from build123d import *

# Parameters (mm, degrees)
BOSS_EXTRUDE1_DEPTH = 5.08
SKETCH3_W           = 12.7
SKETCH3_H           = 12.7
SKETCH3_H_2         = 12.575411903
SKETCH3_W_2         = 12.822150439
CUT_EXTRUDE1_DEPTH  = 114.705788771


with BuildPart() as part:
    # Sketch2 → Boss-Extrude1 (new body)
    with BuildSketch(Plane(origin=(0, 0, 0), x_dir=(1, 0, 0), z_dir=(0, 1, 0))):
        with BuildLine():
            Line((-88.9, -50.8), (88.9, -50.8))
            ThreePointArc((88.9, -50.8), (97.880256121, -47.080256121), (101.6, -38.1))
            Line((101.6, -38.1), (101.6, 38.1))
            ThreePointArc((101.6, 38.1), (97.880256121, 47.080256121), (88.9, 50.8))
            Line((88.9, 50.8), (-88.9, 50.8))
            ThreePointArc((-88.9, 50.8), (-97.880256121, 47.080256121), (-101.6, 38.1))
            Line((-101.6, 38.1), (-101.6, -38.1))
            ThreePointArc((-101.6, -38.1), (-97.880256121, -47.080256121), (-88.9, -50.8))
        make_face()
    extrude(amount=BOSS_EXTRUDE1_DEPTH)

    # Sketch3 → Cut-Extrude1 (cut, through all)
    with BuildSketch(Plane(origin=(0, 5.08, 0), x_dir=(1, 0, 0), z_dir=(0, 1, 0))):
        with Locations((-69.838651623, -44.45)):
            Rectangle(SKETCH3_W, SKETCH3_H)
        with Locations((-69.838651623, 44.512294049)):
            Rectangle(SKETCH3_W, SKETCH3_H_2)
        with Locations((69.673417763, -44.45)):
            Rectangle(SKETCH3_W_2, SKETCH3_H)
        with Locations((69.673417763, 44.512294049)):
            Rectangle(SKETCH3_W_2, SKETCH3_H_2)
    extrude(amount=-CUT_EXTRUDE1_DEPTH, mode=Mode.SUBTRACT)


solid = part.part
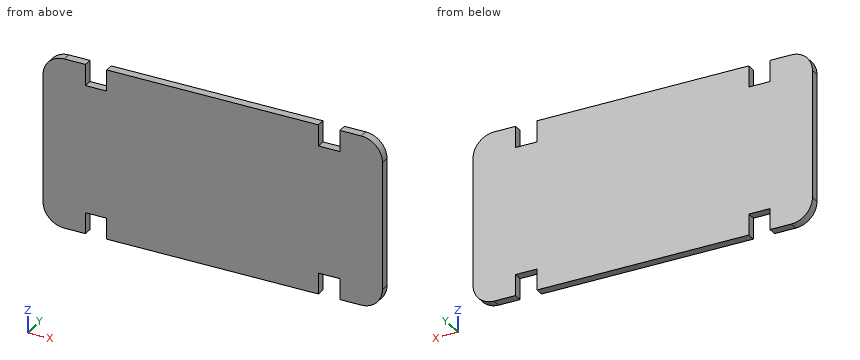
Could you check a few things on this model? Use its own coordinates, in mm. Round coordinates to 2 decimals unless told otherwise and drop trailing zeros. Order: outer loops, then holes, each group sorted by start corner. A loop starts at its lowest first (then second) coordinate and runs counter-clockwise, first axis right, second up.
Q1. Imagine slicing it at B-B, the plane x = 68. List the corners of the cut face in (y, z) for me.
Geometry says:
outline: (0, -38.22) - (5.08, -38.22) - (5.08, 38.1) - (0, 38.1) - close
Q2. Please list where these lines run through material, in increasing order: probe 1 along X at (y, z) = (4.3, -39.5); probe 2 along X at (y, z) = (0.4, 43); probe 3 along Z at (x, y) = (-89.5, 0.6).
Geometry says:
probe 1: x = -101.52 to -76.19, -63.49 to 63.26, 76.08 to 101.52
probe 2: x = -100.62 to -76.19, -63.49 to 63.26, 76.08 to 100.62
probe 3: z = -50.79 to 50.79
Q3. Imagine slicing it at A-A, the plane y = 3.5. List the corners of the cut face in (x, z) for me.
Geometry says:
outline: (-101.6, -38.1) arc R12.7 ccw to (-88.9, -50.8) - (-76.19, -50.8) - (-76.19, -38.22) - (-63.49, -38.22) - (-63.49, -50.8) - (63.26, -50.8) - (63.26, -38.22) - (76.08, -38.22) - (76.08, -50.8) - (88.9, -50.8) arc R12.7 ccw to (101.6, -38.1) - (101.6, 38.1) arc R12.7 ccw to (88.9, 50.8) - (76.08, 50.8) - (76.08, 38.1) - (63.26, 38.1) - (63.26, 50.8) - (-63.49, 50.8) - (-63.49, 38.1) - (-76.19, 38.1) - (-76.19, 50.8) - (-88.9, 50.8) arc R12.7 ccw to (-101.6, 38.1) - close
Q4. I'm going to push flat-ended pins straight in: P1, Ø2.5, axis at y = 1.5, z = -42.5, coming from the -X side; P2, Ø1.5, axis at y = 1.5, z = -45, coming from the +X side; P3, Ø1.5, axis at y = 2, z = 41.5, coming from the -X side; P4, Ø5, axis at x = 52.5, z = 38.5, coming from the -Y side. Where does each tip first touch, or does it pass through?
Geometry says:
P1: stops at x = -101.2
P2: stops at x = 100.01
P3: stops at x = -101.32
P4: stops at y = 0
